Verification items for the finished model (mm, model axes). Face numbers are marked on the shaded views. Round coordinates to 2 decimals unless told otherwise and drop trailing zeros. Write each loop counter-clockwise with the first axis right and the second up, starting at its lowest first coordinate (ties: lowest second). Pieces come first, ordered by that corner, then holes. Notation, with made-up numbers: (-33.5, 77) - (0.5, 77) arc R31 cw to (0.5, 106) - close; hole circle Ø5 at (87, -4.5). An arc over 180 degrees is marked (long way). Answer as a JSON object with one key per item and string values. Group by question number.
1) Section check C-C (y = 0). Enter the section's corners in (x, z), then the cut area to 3 significant figures.
2) Thickness scan on line 1 (X direction, y = 0, z = 3.7); line 2 (Y direction, x = 0, z = 2.45); line 3 (X direction, y = 0, z = 2.3). Record the ranges inside material, lowest first.
3) Section check A-A (x = 0). Enter the section's corners in (y, z).
4) Go/stop test with flat-tipped pins: pin 1 Ø1.4 at (y, z) = (20.5, 1.5) entering from -X; pin 2 Ø1.1 at (y, z) = (3, 4) entering from +X; pin 3 Ø2.5 at (x, y) = (0, 21.5) entering from +Z; pin 4 Ø1.4 at (y, z) = (21, 1.5) entering from +X. Record where each tip stops, or that it passes through.
5) Mould release check, pull along X, two halves, no side actions. Record for the marked faces 1, 2 and 3: +X half, -X half, draft (parallel to the pull), parting line (faces both ways), or undercut.
6) Section check D-D (y = 22). Enter the section's corners in (x, z), then the cut area to 3 significant figures.
7) Section check B-B (z = 1.9). Enter the section's corners in (x, y).
```python
from build123d import *

# Parameters (mm, degrees)
EXTRUDE_DEPTH = 3.3
SKETCH001_R   = 1.5
POCKET_DEPTH  = 3.301
PAD_DEPTH     = 1


with BuildPart() as part:
    # Sketch → Extrude (new body)
    with BuildSketch(Plane.XY):
        with BuildLine():
            ThreePointArc((3.5, 21.5), (0, 25), (-3.5, 21.5))
            Line((-3.5, 21.5), (-3.5, 19.691369))
            ThreePointArc((-3.5, 19.691369), (0, -20), (3.5, 19.691369))
            Line((3.5, 19.691369), (3.5, 21.5))
        make_face()
    extrude(amount=EXTRUDE_DEPTH)

    # Sketch001 → Pocket (cut, through all)
    with BuildSketch(Plane.XY.offset(3.3)):
        with Locations((0, 21.5)):
            Circle(SKETCH001_R)
    extrude(amount=-POCKET_DEPTH, mode=Mode.SUBTRACT)

    # Sketch002 → Pad (new body)
    with BuildSketch(Plane.XY.offset(3.3)):
        with BuildLine():
            ThreePointArc((-4.5, 7.022984), (0, -8.341002), (4.5, 7.022984))
            Line((4.5, 11.124298), (4.5, 7.022984))
            ThreePointArc((-4.5, 11.124298), (0, -12), (4.5, 11.124298))
            Line((-4.5, 7.022984), (-4.5, 11.124298))
        make_face()
        with BuildLine():
            ThreePointArc((1.5, 14.356668), (0, 15.856668), (-1.5, 14.356668))
            Line((-1.5, 14.356668), (-1.5, -4.143332))
            ThreePointArc((-1.5, -4.143332), (0, -5.643332), (1.5, -4.143332))
            Line((1.5, 14.356668), (1.5, -4.143332))
        make_face()
    extrude(amount=PAD_DEPTH)


solid = part.part
```
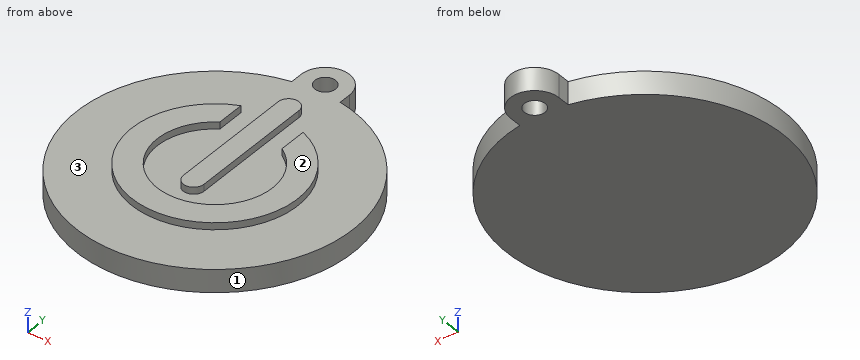
Returned:
{
 "1": {"outline": "(-20, 0) - (20, 0) - (20, 3.3) - (12, 3.3) - (12, 4.3) - (8.34, 4.3) - (8.34, 3.3) - (1.5, 3.3) - (1.5, 4.3) - (-1.5, 4.3) - (-1.5, 3.3) - (-8.34, 3.3) - (-8.34, 4.3) - (-12, 4.3) - (-12, 3.3) - (-20, 3.3) - close", "area": "142 mm2"},
 "2": {"line 1": "-12 to -8.34, -1.5 to 1.5, 8.34 to 12", "line 2": "-20 to 20, 23 to 25", "line 3": "-20 to 20"},
 "3": {"outline": "(-20, 0) - (20, 0) - (20, 3.3) - (15.86, 3.3) - (15.86, 4.3) - (-5.64, 4.3) - (-5.64, 3.3) - (-8.34, 3.3) - (-8.34, 4.3) - (-12, 4.3) - (-12, 3.3) - (-20, 3.3) - close; (23, 0) - (25, 0) - (25, 3.3) - (23, 3.3) - close"},
 "4": {"pin 1": "x = -3.5", "pin 2": "x = 11.75", "pin 3": "through", "pin 4": "x = 3.5"},
 "5": {"face 1": "parting line", "face 2": "draft", "face 3": "undercut"},
 "6": {"outline": "(-3.46, 0) - (-1.41, 0) - (-1.41, 3.3) - (-3.46, 3.3) - close; (1.41, 0) - (3.46, 0) - (3.46, 3.3) - (1.41, 3.3) - close", "area": "13.5 mm2"},
 "7": {"outline": "(-3.5, 19.69) arc R20 ccw (long way) to (3.5, 19.69) - (3.5, 21.5) arc R3.5 ccw to (-3.5, 21.5) - close; hole circle Ø3 at (0, 21.5)"}
}
